from build123d import *

# Parameters (mm, degrees)
BOSS_EXTRUDE1_START = -2
SKETCH1_R           = 0.8
BOSS_EXTRUDE1_DEPTH = 1.5


with BuildPart() as part:
    # Sketch1 → Boss-Extrude1 (new body)
    with BuildSketch(Plane.XY.offset(BOSS_EXTRUDE1_START)):
        with BuildLine():
            Line((7.571676853, 3.903865442), (6.416086079, 3.903865442))
            Line((6.416086079, 3.903865442), (-6.281037731, 3.903865442))
            Line((-6.281037731, 3.903865442), (-7.609270418, 3.903865442))
            add(Edge.make_bspline(
                [(-7.95528082, 2.295104415), (-7.850615408, 2.833585734), (-7.745718452, 3.376152559), (-7.609270418, 3.903865442)],
                knots=[0.598753878, 0.598753878, 0.598753878, 0.598753878, 0.708182049, 0.708182049, 0.708182049, 0.708182049], degree=3))
            add(Edge.make_bspline(
                [(-8.491604222, -2.143861632), (-8.497541628, -1.753055168), (-8.461188827, -0.260180468), (-8.197652692, 1.215784612), (-7.95528082, 2.295104415)],
                knots=[0.5931491, 0.5931491, 0.5931491, 0.5931491, 0.658813679, 0.84412355, 0.84412355, 0.84412355, 0.84412355], degree=3))
            Line((-8.491604222, -2.143861632), (-10.735900357, -3.15355335))
            Line((-10.735900357, -3.15355335), (-9.505051186, -5.889428039))
            Line((-9.505051186, -5.889428039), (-6.464679246, -4.521557259))
            add(Edge.make_bspline(
                [(-6.464679246, -4.521557259), (-4.951547414, -6.675350117), (-2.029321492, -7.287998666)],
                knots=[0.510655247, 0.510655247, 0.510655247, 1.302217681, 1.302217681, 1.302217681], degree=2, weights=[1, 0.922695664, 1]))
            Line((-2.029321492, -7.287998666), (2.191128147, -7.117218369))
            add(Edge.make_bspline(
                [(2.191128147, -7.117218369), (4.720940331, -6.365516028), (6.056108453, -4.433151977)],
                knots=[1.895445663, 1.895445663, 1.895445663, 2.606320009, 2.606320009, 2.606320009], degree=2, weights=[1, 0.937494442, 1]))
            Line((6.056108453, -4.433151977), (9.406785059, -5.940595847))
            Line((9.406785059, -5.940595847), (10.637634232, -3.204721158))
            Line((10.637634232, -3.204721158), (8.560362384, -2.270172384))
            add(Edge.make_bspline(
                [(8.560362384, -2.270172384), (8.775779374, 0.923139429), (7.571676853, 3.903865442)],
                knots=[0, 0, 0, 1, 1, 1], degree=2))
        make_face()
        with Locations((8.836663947, -4.039290527)):
            Circle(SKETCH1_R, mode=Mode.SUBTRACT)
        with Locations((-8.934930071, -3.988122724)):
            Circle(SKETCH1_R, mode=Mode.SUBTRACT)
    extrude(amount=-BOSS_EXTRUDE1_DEPTH)


solid = part.part
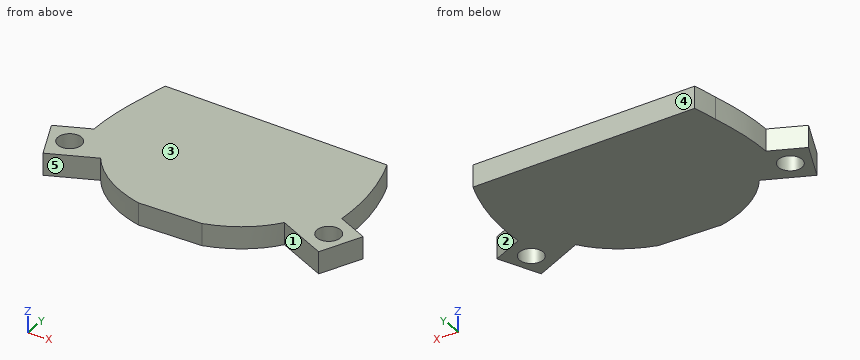
CAD build for the part. Positions are in the model's coordinates, mm. Face numbers are marked on the shaded views. A direction names the side the tool comes from. Round coordinates to 2 decimals unless told otherwise and drop trailing zeros. Loops run counter-clockwise (first coordinate to the right, second up) from the corner with the lowest first, then second, coordinate; pieces in that order, holes last.
(1) Cut at C-C (x = 7.25). Give the cut face in (y, z), plus the area to 3 significant figures.
(2) Cut at A-A (y = -3.75). Give the cut face in (x, z), plus the area to 3 significant figures.
(3) Wall check: line 1 along X through (y, z) = (-5.75, -2.95); line 2 along X through (y, z) = (-5.5, -3.3) (3 decimals); line 3 along Y through (x, z) = (-5, -2.5). Give the ranges that are in metal, low to high.
(4) Two-plate mould, pull along X, no slides. Class the marked faces 1, 2 and 3: +X half, -X half, draft (parallel to the pull), parting line (faces both ways), or undercut.
(5) Which spindle directions (+Z, -Z, +X, -X, +Y, -Y) get a long thin tool onto all of the face, cutting with end or side? Do the marked faces 4 and 5. Say none if no direction does.
(6) Cut at B-B (z = -2.2). State how many separate pieces and enclosed holes the cut face has, plus the area to 3 significant figures.
Findings below:
1. outline: (-4.97, -3.5) - (3.9, -3.5) - (3.9, -2) - (-4.97, -2) - close
1. area: 13.3 mm2
2. outline: (-10.47, -3.5) - (-9.7, -3.5) - (-9.7, -2) - (-10.47, -2) - close; (-8.17, -3.5) - (8.09, -3.5) - (8.09, -2) - (-8.17, -2) - close; (9.58, -3.5) - (10.39, -3.5) - (10.39, -2) - (9.58, -2) - close
2. area: 26.8 mm2
3. line 1: x = -9.57 to -9.2, -5.32 to 4.83, 8.98 to 9.49
3. line 2: x = -9.68 to -8.639, -5.605 to 5.118, 8.427 to 9.605
3. line 3: y = -6 to 3.9
4. face 1: undercut
4. face 2: +X half
4. face 3: draft
5. face 4: +Z, -Z, +X, -X, +Y
5. face 5: +Z, -Z, -Y
6. separate pieces: 1
6. enclosed holes: 2
6. area: 174 mm2
